Here's how the part is built. I have some questions about the finished solid (model axes, mm). A direction names the side the tool comes from. Give positions to 0.01 mm unless a question says otherwise; leave off trailing zeros. Write each loop counter-clockwise with the first axis right and the second up, starting at its lowest first coordinate (ties: lowest second). Pieces come first, ordered by that corner, then holes. Notation, with made-up numbers: (79, -0.75) - (101, -0.75) arc R6 ccw to (101, 9.25) - close; hole circle Ø11 at (42, -35). An arc over 180 degrees is marked (long way). One line per item, written item: value. Start each with the question number.
1) On a 3-axis mill with a long thin cutter (end or side, diameter ignored), from which of +Z, -Z, +X, -X, +Y, -Y can I reach the whole of each face in a straight line? I mean faces 1 (the flat face through (0, -2, 0)), 2 (the cylindrical face through (-0.596, -1.768, -2.685)). Say none if no direction works.
2) I'm going to push flat-ended pins straight in: P1, Ø3, axis at x = -1, y = -9.5, coming from the -Z side; P2, Ø1, axis at y = -5.5, z = 0.5, coming from the -X side; P3, Ø0.8, axis at x = 0.5, z = -0.5, coming from the +Y side. Where does each tip first touch, or does it pass through?
3) Imagine slicing it at B-B on y = -4.75. Write out the boundary of the cut face in (x, z).
4) We'd pull the mould along Z, two halves only. Please class faces 3 (the cylindrical face through (-1.5, -6.8, 0.07)), 4 (the flat face through (1.2, -3, -1.2)), 5 (the flat face through (0.63, -0.99, -1.08)): +Z half, -Z half, draft (parallel to the pull), parting line (faces both ways), or undercut.
5) Please list where these lines run through material, in increasing order: L1, parallel to Y at x = -0.8, z = -1.45; L2, parallel to X at y = -4.5, z = -0.4; L3, parallel to Y at x = -1.8, z = 2. Write a range as [from, to].
6) Imagine slicing it at A-A on z = 0. Write out the boundary of the cut face in (x, y), plus the area to 3 significant figures.
7) Imagine slicing it at C-C on y = -2.5. Write out the boundary of the cut face in (x, z), plus the area to 3 significant figures.
from build123d import *

# Parameters (mm, degrees)
CORTAR_EXTRUIR1_DEPTH = 2
CHAFL_N1_SIZE         = 0.5
REDONDEO1_R           = 0.5


with BuildPart() as part:
    # Croquis1 → Revolución1 (revolve)
    with BuildSketch(Plane.XY):
        Polygon((0, 0), (2.75, 0), (2.75, -3), (1.5, -3), (1.5, -11), (0, -11), align=None)
    revolve(axis=Axis((0, 0, 0), (0, -1, 0)))

    # Croquis2 → Cortar-Extruir1 (cut)
    with BuildSketch(Plane(origin=(0, 0, 0), x_dir=(1, 0, 0), z_dir=(0, 1, 0))):
        Polygon((1.25, 0.721687836), (0, 1.443375673), (-1.25, 0.721687836), (-1.25, -0.721687836), (0, -1.443375673), (1.25, -0.721687836), align=None)
    extrude(amount=-CORTAR_EXTRUIR1_DEPTH, mode=Mode.SUBTRACT)

    # Chaflán1
    chafl_n1_edges = [part.edges().sort_by_distance(p)[0] for p in [
        (-1.5, -11, 0),
    ]]
    chamfer(chafl_n1_edges, length=CHAFL_N1_SIZE)

    # Redondeo1
    redondeo1_edges = [part.edges().sort_by_distance(p)[0] for p in [
        (-2.75, 0, 0),
    ]]
    fillet(redondeo1_edges, radius=REDONDEO1_R)


solid = part.part
Numbers:
1. face 1: +Y
1. face 2: +Y, -Y
2. P1: z = -1.5
2. P2: x = -1.5
2. P3: y = -2
3. outline: circle Ø3 at (0, 0)
4. face 3: parting line
4. face 4: draft
4. face 5: undercut
5. L1: [-3, 0]
5. L2: [-1.45, 1.45]
5. L3: [-3, -0.26]
6. outline: (-2.75, -3) - (-1.5, -3) - (-1.5, -10.5) - (-1, -11) - (1, -11) - (1.5, -10.5) - (1.5, -3) - (2.75, -3) - (2.75, -0.5) arc R0.5 ccw to (2.25, 0) - (1.25, 0) - (1.25, -2) - (-1.25, -2) - (-1.25, 0) - (-2.25, 0) arc R0.5 ccw to (-2.75, -0.5) - close
6. area: 35.1 mm^2
7. outline: circle Ø5.5 at (0, 0)
7. area: 23.8 mm^2
